Source: CAD feature listing. Evaluate the final solid. Frame: model axes, mm. A direction names the side the tool comes from. Give positions to 0.01 mm unless a question says otherwise; leave off trailing zeros. Loops run counter-clockwise (first coordinate to the right, second up) from the corner with the lowest first, then second, coordinate; pieces in that order, holes last. Notation, with made-up numbers: (-10, 58.25) -> (18, 58.25) arc R29 cw to (18, 87.25) -> close; hole circle Ø7 at (38, -19.75). An arc over 180 degrees is marked (long way). Answer as a JSON object with one key per item and string values. Group by question number.
Autodesk Inventor part; units mm, degrees
ref_plane "YZ Plane" through (0, 0, 0) normal (1, 0, 0) x (0, 1, 0)
ref_plane "XZ Plane" through (0, 0, 0) normal (0, 1, 0) x (-1, 0, 0)
ref_plane "XY Plane" through (0, 0, 0) normal (0, 0, 1) x (1, 0, 0)
sketch "Sketch1" plane through (0, 0, 0) normal (0, 0, 1) x (1, 0, 0)
  line L0 (-12.5, 20) -> (12.5, 20)
  line L1 (12.5, 20) -> (12.5, -20)
  line L2 (12.5, -20) -> (-12.5, -20)
  line L3 (-12.5, -20) -> (-12.5, 20)
  point P0 (0, 0)
  point P1 (-12.5, 0)
  point P2 (0, 20)
  dimension "d0" = 40
  dimension "d1" = 25
extrude "Extrusion1" add sketch "Sketch1" along normal blind 15
sketch "Sketch3" plane through (0, 0, 15) normal (0, 0, -1) x (-1, 0, 0)
  line L0 (-12.5, -20) -> (-12.5, 20)
  line L1 (-12.5, -20) -> (-12.5, 20)
  line L2 (12.5, -20) -> (-12.5, -20)
  line L3 (-12.5, 20) -> (12.5, 20)
  line L4 (0, 0) -> (0, 4.9357) construction
  point P0 (-7, -14)
  point P1 (-7, 14)
  point P2 (0, -20)
  point P3 (0, 20)
  point P4 (7, -14)
  point P5 (7, 14)
  dimension "d21" = 6
  dimension "d22" = 6
  dimension "d24" = 5.5
hole "Hole1" at (7, -14, 15) at (-7, -14, 15) at (-7, 14, 15) at (7, 14, 15) direction (0, 0, -1) diameter 5 end through all counterbore diameter 10 counterbore depth 5
sketch "Sketch4" plane through (0, 0, 15) normal (0, 0, 1) x (1, 0, 0)
  line L0 (-12.5, 5) -> (12.5, 5)
  line L1 (12.5, 5) -> (12.5, -5)
  line L2 (12.5, -5) -> (-12.5, -5)
  line L3 (-12.5, -5) -> (-12.5, 5)
  line L4 (12.5, -20) -> (12.5, 20)
  line L5 (-12.5, 20) -> (-12.5, -20)
  point P0 (0, 0)
  point P1 (12.5, 0)
  dimension "d20" = 10
extrude "Extrusion3" add sketch "Sketch4" along normal blind 25
sketch "Sketch5" plane through (-12.5, 5, 15) normal (0, 1, 0) x (1, 0, 0)
  circle A0 centre (10, -13) radius 6
  line L0 (25, -25) -> (0, -25)
  line L1 (25, 0) -> (25, -25)
  circle A1 centre (10, -5) radius 1.75
  circle A2 centre (2, -13) radius 1.75
  circle A3 centre (10, -21) radius 1.75
  circle A4 centre (18, -13) radius 1.75
  point P0 (12.5, 15)
  dimension "d27" = 12
  dimension "d28" = 12
  dimension "d29" = 15
  dimension "d30" = 3.5
  dimension "d31" = 8
  dimension "d34" = 360
extrude "Extrusion4" cut sketch "Sketch5" against normal through all
sketch "Sketch6" plane through (0, 0, 15) normal (0, 0, 1) x (1, 0, 0)
  line L0 (12.5, 5) -> (12.5, 20)
  line L1 (12.5, 9) -> (7, 9)
  circle A0 centre (7, 14) radius 5
  line L2 (2, 20) -> (2, 14)
  line L3 (12.5, 20) -> (-12.5, 20)
  point P0 (0, 0)
  point P1 (12.5, 7)
extrude "Extrusion5" cut sketch "Sketch6" against normal up to surface (5 mm away) contours L1 A0 L2 L3 L0
mirror "Mirror1" about plane through (0, 0, 0) normal (1, 0, 0) of "Extrusion5"
mirror "Mirror2" about plane through (0, 0, 0) normal (0, 1, 0) of "Extrusion5", "Mirror1"
move faces "Move1" translate (-3, 0, 0) faces at (-12.5, 3, 3.3333)
chamfer "Chamfer2" distance 2 angle 45 2 edges at (-1.5, 5, 15) (-1.5, -5, 15)
properties part number "0008-10-013 Supăort Piulita Axa Z"
(1) First-contact query: pin 1 (2.5 mm diameter, centred on y = -17, z = 13.5, fed in from -X); pin 2 (12 mm diameter, centred on x = -5, y = -7, fed in from -Z); pin 3 (4 mm diameter, centred on y = -17, z = 13.5, fed in from +X); pin 4 (6 mm diameter, centred on x = 7, y = -14, fed in from +Z). Flat tips, straight axial feed; report the tip coordinate or a pass-through.
(2) Section query D-D on y = -0.5. Return the cut outline in (x, z), plus the area to 3 significant figures.
(3) Section query A-A on z = 28. Return the cut outline in (x, y), plus the area to 3 significant figures.
(4) Mould query, pull axis Z, two halves, no side actions, for faces 4 (the face through (-2.728, 0.07, 18.265)), 5 (the face through (2, -17, 13)), 6 (the face through (-2, 0, 0)), 7 (the face through (-2, 6, 16)). Classes: pulls with the +Z half, pulls with the -Z half, needs draft (parallel to the pull), parting line crosses it, or undercut.
(5) Material intervals for line 1 (Z direction, x = -2.5, y = -2); line 2 (Y direction, x = -7, z = 2.5); line 3 (X direction, y = 14, z = 6.25), sorted ascending. Write a range as from..to.
(6) Access query for faces 1 (the face through (-11, 9, 13)), 2 (the face through (-1, 12, 15)), 3 (the face through (-4, -10, 12)). Directions: +Z, -Z, +X, -X, +Y, -Y. A direction counts if a zero-diameter tool reaches every point of the face in a straight line with its end or side. Return the directions, or none.
(7) Section query B-B on x = -10.5. Return the cut outline in (y, z), plus the area to 3 significant figures.
(8) Section query C-C on z = 20. Return the cut outline in (x, y), plus the area to 3 significant figures.
Result:
{
 "1": {"pin 1": "x = -2", "pin 2": "z = 0", "pin 3": "x = 2", "pin 4": "z = 10"},
 "2": {"outline": "(-15.5, 0) -> (12.5, 0) -> (12.5, 40) -> (-15.5, 40) -> close; hole circle Ø3.5 at (-10.5, 28); hole circle Ø12 at (-2.5, 28); hole circle Ø3.5 at (-2.5, 20); hole circle Ø3.5 at (-2.5, 36); hole circle Ø3.5 at (5.5, 28)", "area": "968 mm²"},
 "3": {"outline": "(-15.5, -5) -> (-12.25, -5) -> (-12.25, 5) -> (-15.5, 5) -> close; (-8.75, -5) -> (-8.5, -5) -> (-8.5, 5) -> (-8.75, 5) -> close; (3.5, -5) -> (3.75, -5) -> (3.75, 5) -> (3.5, 5) -> close; (7.25, -5) -> (12.5, -5) -> (12.5, 5) -> (7.25, 5) -> close", "area": "90.0 mm²"},
 "4": {"face 4": "undercut", "face 5": "needs draft", "face 6": "pulls with the -Z half", "face 7": "pulls with the +Z half"},
 "5": {"line 1": "0..18.25, 21.75..22, 34..34.25, 37.75..40", "line 2": "-20..-16.5, -11.5..11.5, 16.5..20", "line 3": "-15.5..-9.5, -4.5..4.5, 9.5..12.5"},
 "6": {"face 1": "+Z, -X, +Y", "face 2": "+Z, +X, -X, +Y", "face 3": "+Z, -X, -Y"},
 "7": {"outline": "(-20, 0) -> (20, 0) -> (20, 10) -> (9, 10) -> (9, 15) -> (7, 15) -> (5, 17) -> (5, 26.25) -> (-5, 26.25) -> (-5, 17) -> (-7, 15) -> (-9, 15) -> (-9, 10) -> (-20, 10) -> close; (-5, 29.75) -> (5, 29.75) -> (5, 40) -> (-5, 40) -> close", "area": "709 mm²"},
 "8": {"outline": "(-15.5, -5) -> (-4.25, -5) -> (-4.25, 5) -> (-15.5, 5) -> close; (-0.75, -5) -> (12.5, -5) -> (12.5, 5) -> (-0.75, 5) -> close", "area": "245 mm²"}
}
